Part model, mm, in its own coordinate system. Give positions to 0.01 mm unless a question says otherwise; leave off trailing zeros. Write each loop counter-clockwise with the first axis right and the second up, starting at its lowest first coordinate (ties: lowest second). Pieces come first, ordered by that corner, then holes.
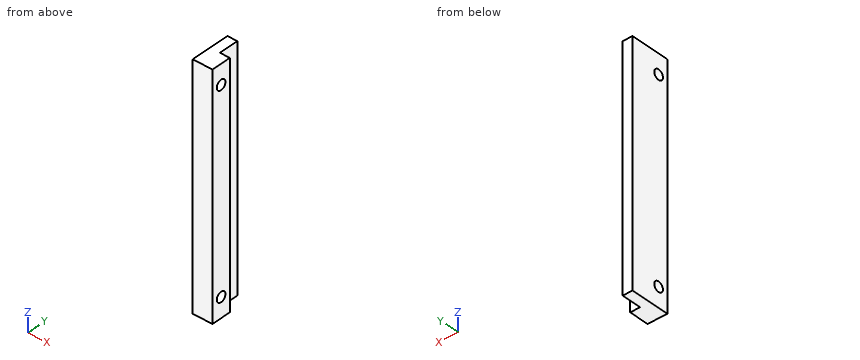
```python
from build123d import *

# Parameters (mm, degrees)
BOSS_EXTRUDE1_DEPTH     = 76.2
SKETCH2_R               = 3.175
CUT_EXTRUDE1_DEPTH      = 1
CUT_EXTRUDE1_DEPTH_BACK = 13.7


with BuildPart() as part:
    # Sketch1 → Boss-Extrude1 (new body, symmetric)
    with BuildSketch(Plane.XY):
        Polygon((0, 12.7), (0, 0), (6.35, 0), (6.35, -12.7), (-6.35, -12.7), (-6.35, 12.7), align=None)
    extrude(amount=BOSS_EXTRUDE1_DEPTH, both=True)

    # Sketch2 → Cut-Extrude1 (cut, two sides)
    with BuildSketch(Plane.ZY.offset(6.35)) as cut_extrude1_sk:
        with Locations((-63.5, -6.35)):
            Circle(SKETCH2_R)
        with Locations((63.5, -6.35)):
            Circle(SKETCH2_R)
    extrude(amount=CUT_EXTRUDE1_DEPTH, mode=Mode.SUBTRACT)
    extrude(cut_extrude1_sk.sketch, amount=-CUT_EXTRUDE1_DEPTH_BACK, mode=Mode.SUBTRACT)


solid = part.part
```
1) Saw through at B-B, the plane y = -6.35. Write the cut outline in (x, z) (3 decimals), then the cut area to 3 significant figures.
Answers follow:
outline: (-6.35, -76.2) - (6.35, -76.2) - (6.35, -66.675) - (-6.35, -66.675) - close; (-6.35, -60.325) - (6.35, -60.325) - (6.35, 60.325) - (-6.35, 60.325) - close; (-6.35, 66.675) - (6.35, 66.675) - (6.35, 76.2) - (-6.35, 76.2) - close
area: 1,770 mm2
2) Wall check: L1, parallel to Y at x = -0.75, z = -63.5 (3 decimals); L2, parallel to Z at x = 2.25, y = -4.75; L3, parallel to Z at x = 0.5, y = -7. Give the ranges that are in metal, low to high.
Answers follow:
L1: y = -12.7 to -9.525, -3.175 to 12.7
L2: z = -76.2 to -66.24, -60.76 to 60.76, 66.24 to 76.2
L3: z = -76.2 to -66.61, -60.39 to 60.39, 66.61 to 76.2
3) Saw through at A-A, the plane z = 63.5. Write the cut outline in (x, y) (3 decimals).
Answers follow:
outline: (-6.35, -12.7) - (6.35, -12.7) - (6.35, -9.525) - (-6.35, -9.525) - close; (-6.35, -3.175) - (6.35, -3.175) - (6.35, 0) - (0, 0) - (0, 12.7) - (-6.35, 12.7) - close
4) Pin check, flat tips, straight feed: pin 1 Ø4 at (y, z) = (-6.35, -63.5) entering from -X; pin 2 Ø1.9 at (x, z) = (2.5, -6.5) entering from +Y; pin 3 Ø6.5 at (y, z) = (9, -24) entering from +X. Stop position of each tip, or through.
Answers follow:
pin 1: passes through
pin 2: stops at y = 0
pin 3: stops at x = 0
5) Saw through at D-D, the plane y = 8.5. Write the cut outline in (x, z), then the cut area to 3 significant figures.
Answers follow:
outline: (-6.35, -76.2) - (0, -76.2) - (0, 76.2) - (-6.35, 76.2) - close
area: 968 mm2
6) Saw through at C-C, the plane x = 2. Write the cut outline in (y, z) (3 decimals).
Answers follow:
outline: (-12.7, -76.2) - (0, -76.2) - (0, 76.2) - (-12.7, 76.2) - close; hole circle Ø6.35 at (-6.35, -63.5); hole circle Ø6.35 at (-6.35, 63.5)
